from build123d import *

# Parameters (mm, degrees)
SKETCH1_W           = 140
SKETCH1_H           = 70
BOSS_EXTRUDE1_DEPTH = 10
BOSS_EXTRUDE2_DEPTH = 25
FILLET2_R           = 16
FILLET1_R           = 3


with BuildPart() as part:
    # Sketch1 → Boss-Extrude1 (new body)
    with BuildSketch(Plane(origin=(0, 0, 0), x_dir=(1, 0, 0), z_dir=(0, 1, 0))):
        with Locations((70, 35)):
            Rectangle(SKETCH1_W, SKETCH1_H)
    extrude(amount=BOSS_EXTRUDE1_DEPTH)

    # Sketch2 → Boss-Extrude2 (add)
    with BuildSketch(Plane(origin=(0, 10, 0), x_dir=(1, 0, 0), z_dir=(0, 1, 0))):
        with BuildLine():
            ThreePointArc((52.5, 35), (52.45506934, 36.253217594), (52.320508076, 37.5))
            Line((52.320508076, 37.5), (47.247448714, 37.5))
            ThreePointArc((47.247448714, 37.5), (47.436701913, 36.256362025), (47.5, 35))
            ThreePointArc((47.5, 35), (47.436701913, 33.743637975), (47.247448714, 32.5))
            Line((47.247448714, 32.5), (52.320508076, 32.5))
            ThreePointArc((52.320508076, 32.5), (52.45506934, 33.746782406), (52.5, 35))
        make_face()
        with BuildLine():
            Line((47.247448714, 37.5), (52.320508076, 37.5))
            ThreePointArc((52.320508076, 37.5), (17.5, 35), (52.320508076, 32.5))
            Line((52.320508076, 32.5), (47.247448714, 32.5))
            ThreePointArc((47.247448714, 32.5), (22.5, 35), (47.247448714, 37.5))
        make_face()
        with BuildLine():
            Line((70, 32.5), (70, 37.5))
            Line((70, 37.5), (52.320508076, 37.5))
            ThreePointArc((52.320508076, 37.5), (52.45506934, 36.253217594), (52.5, 35))
            ThreePointArc((52.5, 35), (52.45506934, 33.746782406), (52.320508076, 32.5))
            Line((52.320508076, 32.5), (70, 32.5))
        make_face()
        with BuildLine():
            Line((87.679491924, 37.5), (70, 37.5))
            Line((70, 37.5), (70, 32.5))
            Line((70, 32.5), (87.679491924, 32.5))
            ThreePointArc((87.679491924, 32.5), (87.5, 35), (87.679491924, 37.5))
        make_face()
        with BuildLine():
            ThreePointArc((122.5, 35), (106.253217594, 52.45506934), (87.679491924, 37.5))
            Line((87.679491924, 37.5), (92.752551286, 37.5))
            ThreePointArc((92.752551286, 37.5), (106.256362025, 47.436701913), (117.5, 35))
            ThreePointArc((117.5, 35), (106.256362025, 22.563298087), (92.752551286, 32.5))
            Line((92.752551286, 32.5), (87.679491924, 32.5))
            ThreePointArc((87.679491924, 32.5), (106.253217594, 17.54493066), (122.5, 35))
        make_face()
        with BuildLine():
            Line((92.752551286, 37.5), (87.679491924, 37.5))
            ThreePointArc((87.679491924, 37.5), (87.5, 35), (87.679491924, 32.5))
            Line((87.679491924, 32.5), (92.752551286, 32.5))
            ThreePointArc((92.752551286, 32.5), (92.5, 35), (92.752551286, 37.5))
        make_face()
    extrude(amount=BOSS_EXTRUDE2_DEPTH)

    # Fillet2
    fillet2_edges = [part.edges().sort_by_distance(p)[0] for p in [
        (0, 5, -70),
        (140, 5, -70),
        (140, 5, 0),
        (0, 5, 0),
    ]]
    fillet(fillet2_edges, radius=FILLET2_R)

    # Fillet1
    fillet1_edges = [part.edges().sort_by_distance(p)[0] for p in [
        (0, 10, -35),
        (70, 10, -70),
        (70, 10, 0),
        (140, 10, -35),
        (4.686291501, 10, -4.686291501),
        (135.313708499, 10, -4.686291501),
        (135.313708499, 10, -65.313708499),
        (4.686291501, 10, -65.313708499),
    ]]
    fillet(fillet1_edges, radius=FILLET1_R)


solid = part.part
Model file for the job. Use its own axes, mm. A direction names the side the tool comes from. Give positions to 0.01 mm unless a question says otherwise; leave off trailing zeros. Order: outer loops, then holes, each group sorted by start corner. A loop starts at its lowest first (then second) coordinate and runs counter-clockwise, first axis right, second up. Notation, with made-up numbers: (68, 11.25) - (81, 11.25) arc R17 ccw to (81, 34.25) - close; hole circle Ø3 at (16, 72.25). An arc over 180 degrees is marked (long way). One line per item, written item: value.
Item 1: Pin check, flat tips, straight feed: pin 1 Ø12 at (x, y) = (98, 16.5) entering from -Z; pin 2 Ø3 at (y, z) = (17.5, -24.5) entering from +X; pin 3 Ø22.5 at (x, z) = (35, -35) entering from +Y. Stop position of each tip, or through.
Response values:
pin 1: z = -52.47
pin 2: x = 120.01
pin 3: y = 10
Item 2: Slice it at C-C (z = -44). List the corners of the cut face in (x, y).
Response values:
outline: (0, 0) - (140, 0) - (140, 7) arc R3 ccw to (137, 10) - (120.01, 10) - (120.01, 35) - (113.67, 35) - (113.67, 10) - (96.33, 10) - (96.33, 35) - (89.99, 35) - (89.99, 10) - (50.01, 10) - (50.01, 35) - (43.67, 35) - (43.67, 10) - (26.33, 10) - (26.33, 35) - (19.99, 35) - (19.99, 10) - (3, 10) arc R3 ccw to (0, 7) - close
Item 3: Wall check: line 1 (Z direction, x = 35, y = 17.5); line 2 (X direction, y = 22.5, z = -30.5); line 3 (X direction, y = 21, z = -27). Give the ranges that are in metal, low to high.
Response values:
line 1: -52.5 to -47.5, -22.5 to -17.5
line 2: 18.09 to 23.34, 46.66 to 51.91, 88.09 to 93.34, 116.66 to 121.91
line 3: 19.44 to 25.4, 44.6 to 50.56, 89.44 to 95.4, 114.6 to 120.56
Item 4: Slice it at A-A (y = 15). List the corners of the cut face in (x, z), then the cut area to 3 significant figures.
Response values:
outline: (52.32, -37.5) - (87.68, -37.5) arc R17.5 ccw (long way) to (87.68, -32.5) - (52.32, -32.5) arc R17.5 ccw (long way) to start; hole circle Ø25 at (35, -35); hole circle Ø25 at (105, -35)
area: 1,120 mm2
Item 5: Tool access for faces 1 (the flat face through (70, 22, -32.5)), 2 (the flat face through (70, 22, -37.5)), 3 (the cylindrical face through (17.515, 22.325, -35.734)), 4 (the flat face through (70, 35, -36)): list every direction of +Z, -Z, +X, -X, +Y, -Y with a clear straight run to the whole face (end or side of a thin tool).
Response values:
face 1: +Z, +Y
face 2: -Z, +Y
face 3: +Y
face 4: +Z, -Z, +X, -X, +Y
Item 6: Slice it at B-B (x = 55.5). List the corners of the cut face in (y, z).
Response values:
outline: (0, -70) - (7, -70) arc R3 ccw to (10, -67) - (10, -37.5) - (35, -37.5) - (35, -32.5) - (10, -32.5) - (10, -3) arc R3 ccw to (7, 0) - (0, 0) - close
Item 7: Slice it at D-D (y = 5.5). List the corners of the cut face in (x, z).
Response values:
outline: (0, -54) arc R16 ccw to (16, -70) - (124, -70) arc R16 ccw to (140, -54) - (140, -16) arc R16 ccw to (124, 0) - (16, 0) arc R16 ccw to (0, -16) - close
Item 8: Two-plate mould, pull along X, no slides. Class faces 5 (the cylindrical face through (139.14, 9.1, -34.73)), 6 (the flat face through (69, 3, 0)), 7 (the cylindrical face through (4.563, 3.549, -4.811)), 8 (the flat face through (105, 10, -35)): released by +X, released by -X, zero draft, split by the parting line, or undercut.
Response values:
face 5: released by +X
face 6: zero draft
face 7: released by -X
face 8: undercut
